```python
from build123d import *

# Parameters (mm, degrees)
SKETCH1_R           = 11
SKETCH1_R_2         = 5
SKETCH1_R_3         = 1.5
BOSS_EXTRUDE1_DEPTH = 2
SKETCH1_3_R         = 5
BOSS_EXTRUDE2_DEPTH = 12
SKETCH2_R           = 1.5
CUT_EXTRUDE1_DEPTH  = 10


with BuildPart() as part:
    # Sketch1 → Boss-Extrude1 (new body)
    with BuildSketch(Plane(origin=(0, 0, 0), x_dir=(1, 0, 0), z_dir=(0, 1, 0))):
        Circle(SKETCH1_R)
        Circle(SKETCH1_R_2, mode=Mode.SUBTRACT)
        with Locations((8, 0)):
            Circle(SKETCH1_R_3, mode=Mode.SUBTRACT)
        with Locations((0, -8)):
            Circle(SKETCH1_R_3, mode=Mode.SUBTRACT)
        with Locations((-8, 0)):
            Circle(SKETCH1_R_3, mode=Mode.SUBTRACT)
        with Locations((0, 8)):
            Circle(SKETCH1_R_3, mode=Mode.SUBTRACT)
    extrude(amount=BOSS_EXTRUDE1_DEPTH)

    # Sketch1_3 → Boss-Extrude2 (add)
    with BuildSketch(Plane(origin=(0, 0, 0), x_dir=(1, 0, 0), z_dir=(0, 1, 0))):
        Circle(SKETCH1_3_R)
    extrude(amount=BOSS_EXTRUDE2_DEPTH)

    # Sketch2 → Cut-Extrude1 (cut)
    with BuildSketch(Plane(origin=(0, 12, 0), x_dir=(1, 0, 0), z_dir=(0, 1, 0))):
        Circle(SKETCH2_R)
    extrude(amount=-CUT_EXTRUDE1_DEPTH, mode=Mode.SUBTRACT)


solid = part.part
```
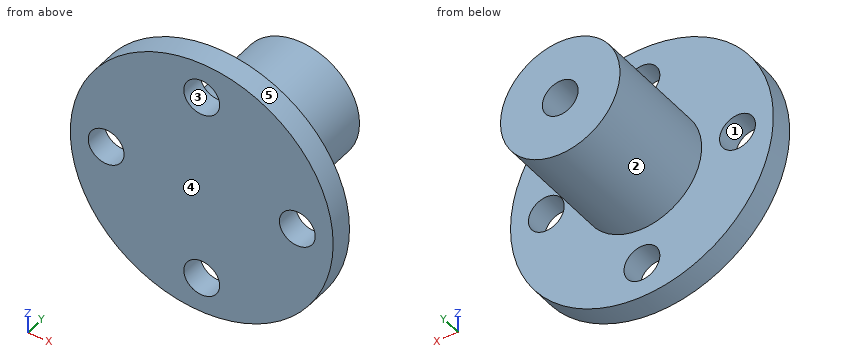
Can you work these out from the model? Positions are in its coordinate system, mm. Face numbers are marked on the shaded views. A direction names the side the tool comes from. Coordinates: 2 decimals unless noted, no trailing zeros. Order: outer loops, then holes, each group sorted by start corner. A loop starts at its lowest first (then second) coordinate and runs counter-clockwise, first axis right, second up.
1. I'm going to push flat-ended pins straight in: pin 1 (4 mm diameter, centred on x = 8, z = 0, fed in from +Y); pin 2 (6 mm diameter, centred on x = 5.5, y = 10, fed in from -Z); pin 3 (4 mm diameter, centred on y = 10.5, z = 2.5, fed in from -X); pin 4 (2.5 mm diameter, centred on x = 0, z = -8, fed in from -Y). Where does each tip first touch, or does it pass through?
2. If we section it at D-D (x = -8): Please give me the cut outline in (y, z), then the cut area to 3 significant figures.
3. Thinking about a two-plate mould opening in X: for the marked faces 3, 4 and 5, which applies, +X half, -X half, draft (parallel to the pull), parting line (faces both ways), or undercut?
4. For the marked faces 1 and 2, which set-ups out of +Z, -Z, +X, -X, +Y, -Y let a thin tool reach every point of the face, with its end or its side?
5. If we section it at B-B (x = 0): Please give me the cut outline in (y, z).
6. If we section it at C-C (y = 0.5): Please give me the cut outline in (x, z), then the cut area to 3 significant figures.
7. I need wall thicknesses on line 1 (Z direction, x = 0, y = 1.45); line 2 (Z direction, x = 0, y = 6.5); line 3 (Y direction, x = 5, z = -9.5). Which ranges of each line are inside material? Lowest first, please.
8. If we section it at A-A (z = 0): Please give me the cut outline in (x, y).
Entries:
1. pin 1: stops at y = 2
1. pin 2: stops at z = -4.33
1. pin 3: stops at x = -4.97
1. pin 4: passes through
2. outline: (0, -7.55) - (2, -7.55) - (2, -1.5) - (0, -1.5) - close; (0, 1.5) - (2, 1.5) - (2, 7.55) - (0, 7.55) - close
2. area: 24.2 mm2
3. face 3: undercut
3. face 4: draft
3. face 5: parting line
4. face 1: +Y, -Y
4. face 2: +Y
5. outline: (0, -11) - (2, -11) - (2, -9.5) - (0, -9.5) - close; (0, -6.5) - (2, -6.5) - (2, -5) - (12, -5) - (12, -1.5) - (2, -1.5) - (2, 1.5) - (12, 1.5) - (12, 5) - (2, 5) - (2, 6.5) - (0, 6.5) - close; (0, 9.5) - (2, 9.5) - (2, 11) - (0, 11) - close
6. outline: circle Ø22 at (0, 0); hole circle Ø3 at (-8, 0); hole circle Ø3 at (0, -8); hole circle Ø3 at (0, 8); hole circle Ø3 at (8, 0)
6. area: 352 mm2
7. line 1: z = -11 to -9.5, -6.5 to 6.5, 9.5 to 11
7. line 2: z = -5 to -1.5, 1.5 to 5
7. line 3: y = 0 to 2
8. outline: (-11, 0) - (-9.5, 0) - (-9.5, 2) - (-11, 2) - close; (-6.5, 0) - (6.5, 0) - (6.5, 2) - (5, 2) - (5, 12) - (1.5, 12) - (1.5, 2) - (-1.5, 2) - (-1.5, 12) - (-5, 12) - (-5, 2) - (-6.5, 2) - close; (9.5, 0) - (11, 0) - (11, 2) - (9.5, 2) - close
